Geometry check sheet. Reference: the model listing, model coordinates, mm. A direction names the side the tool comes from. Coordinates: 2 decimals unless noted, no trailing zeros. Write each loop counter-clockwise with the first axis right and the second up, starting at its lowest first coordinate (ties: lowest second). Pieces come first, ordered by that corner, then holes. Notation, with made-up numbers: (38, -10) -> (81, -10) arc R8 ccw to (81, 5) -> close; hole circle Ø7 at (33.5, -31.75). An arc over 180 degrees is marked (long way). Answer as CSV lines item,"result".
```python
from build123d import *

# Parameters (mm, degrees)
F0_R           = 41.275
F1_DEPTH       = 476.25
F3_R           = 28.575
F4_DEPTH       = 41.148
F1_FACE_R      = 41.275
F4_FACE_R      = 28.575
F9_D           = 12.7
F9_DEPTH       = 38.1
F9_TIP         = 3.8154649308
F9_ON_F7_D     = 12.7
F9_ON_F7_DEPTH = 38.1
F9_ON_F7_TIP   = 3.8154649308


with BuildPart() as f1:
    # F0 (on Right) → F1 (new body, symmetric)
    with BuildSketch(Plane.YZ):
        Circle(F0_R)
    extrude(amount=F1_DEPTH, both=True)



with BuildPart() as f4:
    # F3 (on offset) → F4 (new body)
    with BuildSketch(Plane.YZ.offset(638.175)):
        Circle(F3_R)
    extrude(amount=-F4_DEPTH)


with BuildPart() as f1_1:
    add(f1.part)

    add(f4.part)  # F5 merges F4
    # F1_face (on face) → F5 section 0
    with BuildSketch(Plane.YZ.offset(476.25)):
        Circle(F1_FACE_R)
    # F4_face (on face) → F5 section 1
    with BuildSketch(Plane(origin=(597.027, 0, 0), x_dir=(0, 1, 0), z_dir=(-1, 0, 0))):
        Circle(F4_FACE_R)
    loft()

    # F6: F1 across plane


with BuildPart() as f1_2:
    add(f1_1.part)
    add(f1_1.part.mirror(Plane.YZ))

    # F9
    with Locations(Plane(origin=(-638.175, 0, 0), x_dir=(0, -1, 0), z_dir=(-1, 0, 0))):
        with Locations((0, 0)):
            Hole(F9_D / 2, depth=F9_DEPTH)
            with Locations((0, 0, -(F9_DEPTH + F9_TIP / 2))):  # 118° drill point
                Cone(0, F9_D / 2, F9_TIP, mode=Mode.SUBTRACT)

    # F9 on F7
    with Locations(Plane.YZ.offset(638.175)):
        with Locations((0, 0)):
            Hole(F9_ON_F7_D / 2, depth=F9_ON_F7_DEPTH)
            with Locations((0, 0, -(F9_ON_F7_DEPTH + F9_ON_F7_TIP / 2))):  # 118° drill point
                Cone(0, F9_ON_F7_D / 2, F9_ON_F7_TIP, mode=Mode.SUBTRACT)


solid = f1_2.part
```
Item 1: Set-up check for faces 1 (the cylindrical face through (617.889, -28.547, 1.256)), 2 (the cylindrical face through (-617.889, -28.547, 1.256)), 3 (the flat face through (-638.175, 0, 7)): record each of +Z, -Z, +X, -X, +Y, -Y from which the full face is reachable in a straight line by a thin tool's end or side.
Responses:
face 1,"+X"
face 2,"-X"
face 3,"+Z, -Z, -X, +Y, -Y"
Item 2: Cross-section at A-A, the plane x = 369.5. Record the cut outline in (y, z) (3 decimals), plus the area to 3 significant figures.
Responses:
outline,"circle Ø82.55 at (0, 0)"
area,"5,350 mm2"
Item 3: Depth check by flat-ended pin: pin 1 Ø5 at (x, z) = (213, -11) entering from +Y; pin 2 Ø12 at (x, y) = (86, 19) entering from +Z; pin 3 Ø2 at (x, y) = (-184.5, 5.5) entering from +Z. Enter the tip coordinate at first touch or a pass-through.
Responses:
pin 1,"stops at y = 40.39"
pin 2,"stops at z = 39.17"
pin 3,"stops at z = 41.03"
Item 4: Cross-section at B-B, the plane x = 544. Record the cut outline in (y, z), plus the area to 3 significant figures.
Responses:
outline,"circle Ø68.3 at (0, 0)"
area,"3,660 mm2"
Item 5: Thickness scan on probe 1 along Z at (x, y) = (613, 0) (3 decimals); probe 2 along Y at (x, z) = (-279.5, -1); probe 3 along Y at (x, z) = (-191.5, 24). Record the ranges inside material, lowest first.
Responses:
probe 1,"z = -28.575 to -6.35, 6.35 to 28.575"
probe 2,"y = -41.26 to 41.26"
probe 3,"y = -33.58 to 33.58"
